Could you check a few things on this model? Use its own coordinates, in mm. A direction names the side the tool comes from. Give positions to 0.01 mm unless a question says otherwise; leave off trailing zeros. Write each loop counter-clockwise with the first axis right and the second up, starting at its lowest first coordinate (ties: lowest second). Pieces come first, ordered by that corner, then holes. Notation, with made-up numbers: (84, 41) - (121, 41) arc R30 ccw to (121, 64) - close; hole circle Ø11 at (21, 18). An arc over 180 degrees is marked (long way). Answer in a Markdown table with one row per item.
from build123d import *

# Parameters (mm, degrees)
SKETCH1_W           = 126
SKETCH1_H           = 102
SKETCH1_R           = 11
SKETCH1_W_2         = 3
SKETCH1_H_2         = 15
SKETCH1_W_3         = 15
SKETCH1_H_3         = 3
BOSS_EXTRUDE1_DEPTH = 8


with BuildPart() as part:
    # Sketch1 → Boss-Extrude1 (new body)
    with BuildSketch(Plane.XY):
        with Locations((12, 0)):
            Rectangle(SKETCH1_W, SKETCH1_H)
        with Locations((-24.15725, 0)):
            Circle(SKETCH1_R, mode=Mode.SUBTRACT)
        with Locations((24.15725, 0)):
            Circle(SKETCH1_R, mode=Mode.SUBTRACT)
        with Locations((-46.5, -35.5)):
            Rectangle(SKETCH1_W_2, SKETCH1_H_2, mode=Mode.SUBTRACT)
        with Locations((-46.5, 35.5)):
            Rectangle(SKETCH1_W_2, SKETCH1_H_2, mode=Mode.SUBTRACT)
        with Locations((70.5, 35.5)):
            Rectangle(SKETCH1_W_2, SKETCH1_H_2, mode=Mode.SUBTRACT)
        with Locations((70.5, -35.5)):
            Rectangle(SKETCH1_W_2, SKETCH1_H_2, mode=Mode.SUBTRACT)
        with Locations((-35.5, 46.5)):
            Rectangle(SKETCH1_W_3, SKETCH1_H_3, mode=Mode.SUBTRACT)
        with Locations((59.5, 46.5)):
            Rectangle(SKETCH1_W_3, SKETCH1_H_3, mode=Mode.SUBTRACT)
        with Locations((-35.5, -46.5)):
            Rectangle(SKETCH1_W_3, SKETCH1_H_3, mode=Mode.SUBTRACT)
        with Locations((59.5, -46.5)):
            Rectangle(SKETCH1_W_3, SKETCH1_H_3, mode=Mode.SUBTRACT)
    extrude(amount=BOSS_EXTRUDE1_DEPTH)


solid = part.part
1) On a 3-axis mill with a long thin cutter (end or side, diameter ignored), from which of +Z, -Z, +X, -X, +Y, -Y can I reach the whole of each face in a straight line? I mean faces 4 (the face through (-51, -1, 4)), 5 (the face through (59, 45, 4)). Say none if no direction works.
Check values:
| item | result |
|---|---|
| face 4 | +Z, -Z, -X, +Y, -Y |
| face 5 | +Z, -Z |
2) If I drill on line 1 (Y direction, x = 56, z = 3.5); line 2 (X direction, y = 36.5, z = 6.5); line 3 (Y direction, x = -28.5, z = 2), over which ranges is the centre line in solid material (lowest first)?
Check values:
| item | result |
|---|---|
| line 1 | y = -51 to -48, -45 to 45, 48 to 51 |
| line 2 | x = -51 to -48, -45 to 69, 72 to 75 |
| line 3 | y = -51 to -48, -45 to -10.11, 10.11 to 45, 48 to 51 |
3) Imagine slicing it at C-C (y = -33.5). List the corners of the cut face in (x, z) for me.
Check values:
| item | result |
|---|---|
| outline | (-51, 0) - (-48, 0) - (-48, 8) - (-51, 8) - close; (-45, 0) - (69, 0) - (69, 8) - (-45, 8) - close; (72, 0) - (75, 0) - (75, 8) - (72, 8) - close |
4) Imagine slicing it at A-A (y = 0). List the corners of the cut face in (x, z) for me, then the cut area to 3 significant figures.
Check values:
| item | result |
|---|---|
| outline | (-51, 0) - (-35.16, 0) - (-35.16, 8) - (-51, 8) - close; (-13.16, 0) - (13.16, 0) - (13.16, 8) - (-13.16, 8) - close; (35.16, 0) - (75, 0) - (75, 8) - (35.16, 8) - close |
| area | 656 mm2 |
5) Imagine slicing it at D-D (z = 6.25). State how many separate pieces and enclosed holes the cut face has, then the cut area to 3 significant figures.
Check values:
| item | result |
|---|---|
| separate pieces | 1 |
| enclosed holes | 10 |
| area | 11,700 mm2 |
6) Imagine slicing it at B-B (x = 19.5). List the corners of the cut face in (y, z) for me, then the cut area to 3 significant figures.
Check values:
| item | result |
|---|---|
| outline | (-51, 0) - (-9.97, 0) - (-9.97, 8) - (-51, 8) - close; (9.97, 0) - (51, 0) - (51, 8) - (9.97, 8) - close |
| area | 657 mm2 |
7) We'd pull the mould along X, two halves only. Please class faces 1 (the face through (75, -1, 4)), 2 (the face through (11, 1, 0)), 3 (the face through (72, -36, 4)): +X half, -X half, draft (parallel to the pull), parting line (faces both ways), or undercut.
Check values:
| item | result |
|---|---|
| face 1 | +X half |
| face 2 | draft |
| face 3 | undercut |
